Geometry: see drawing. Coordinates: mm, zero at the bounding-box minimum. A direction names the side the tool comes from. Coordinates: 2 decimals unless noted, no trailing zeros. Write each loop counter-clockwise with the first axis right and the second up, starting at its lowest first coordinate (ties: lowest second). Pieces come first, ordered by that corner, then holes.
1) Section query D-D (y = 0.75). Output: boundary loops of the cut face in (x, z), then the cut area to 3 significant figures.
2) Section query C-C (z = 23.75). Output: boundary loops of the cut face in (x, y).
3) Pin query (flat end, axial travel): pin 1 Ø1.8 at (x, y) = (6, 4.5) entering from +Z. Return the tip coordinate at first contact, or that it passes through.
4) Draft query along X for the marked faces 3, 4 and 5. Return one class per face: pulls with the +X half, pulls with the -X half, needs draft (parallel to the pull), parting line crosses it, or undercut.
5) Section query B-B (y = 4.15). Output: boundary loops of the cut face in (x, z), then the cut area to 3 significant figures.
6) Set-up query: the marked faces 1 and 2. Return all of +Z, -Z, +X, -X, +Y, -Y with unobstructed straight access to the full face (end or side cutting, diameter ignored); none if empty.
7) Section query A-A (x = 5). Output: boundary loops of the cut face in (y, z), then the cut area to 4 significant figures.
8) Line query: L1, parallel to Z at x = 5, y = 2.4; L2, parallel to X at y = 4.85, z = 5; L3, parallel to Z at x = 5, y = 3. Output: solid intervals per line, ascending.
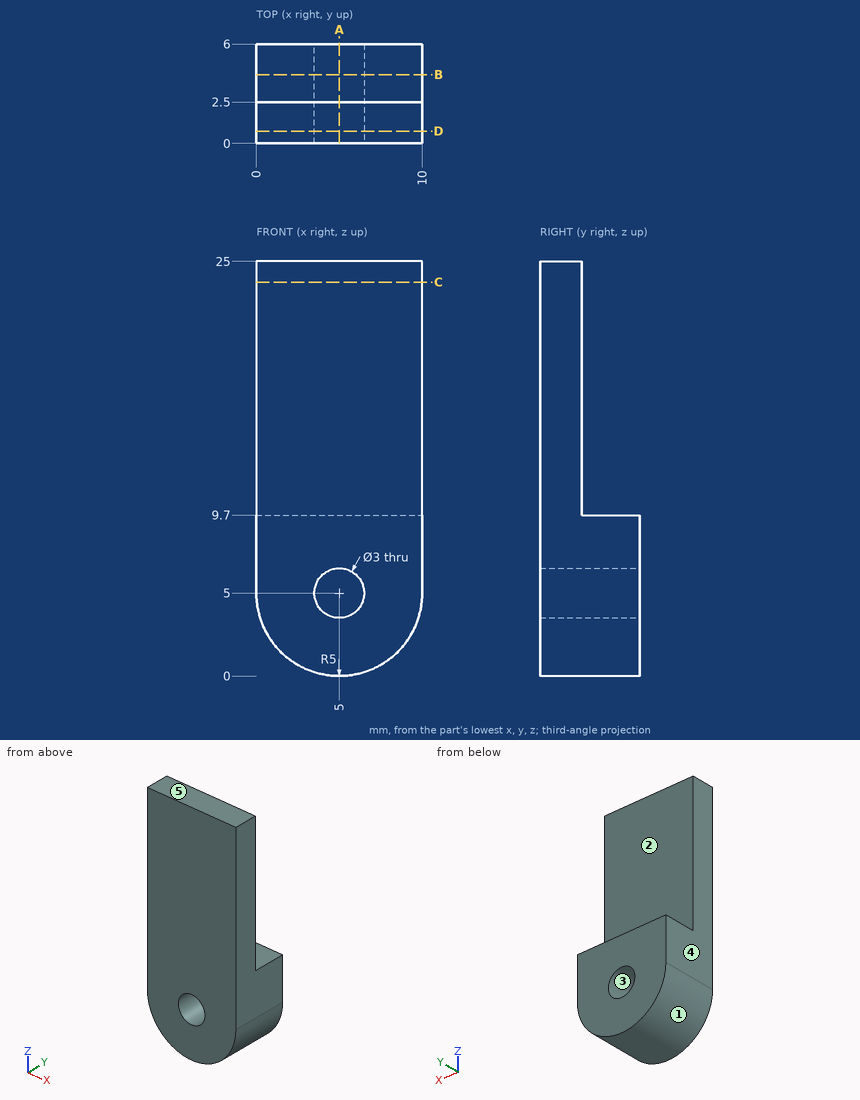
Answer:
1. outline: (0, 5) arc R5 ccw to (10, 5) - (10, 25) - (0, 25) - close; hole circle Ø3 at (5, 5)
1. area: 232 mm2
2. outline: (0, 0) - (10, 0) - (10, 2.5) - (0, 2.5) - close
3. pin 1: stops at z = 9.7
4. face 3: undercut
4. face 4: pulls with the -X half
4. face 5: needs draft
5. outline: (0, 5) arc R5 ccw to (10, 5) - (10, 9.7) - (0, 9.7) - close; hole circle Ø3 at (5, 5)
5. area: 79.2 mm2
6. face 1: -Z, +Y, -Y
6. face 2: +Z, +X, -X, +Y
7. outline: (0, 0) - (6, 0) - (6, 3.5) - (0, 3.5) - close; (0, 6.5) - (6, 6.5) - (6, 9.7) - (2.5, 9.7) - (2.5, 25) - (0, 25) - close
7. area: 78.45 mm2
8. L1: z = 0 to 3.5, 6.5 to 25
8. L2: x = 0 to 3.5, 6.5 to 10
8. L3: z = 0 to 3.5, 6.5 to 9.7
